The listing builds one solid part. Answer for the finished solid, in the listing's coordinates (mm). A direction names the side the tool comes from. Give positions to 0.01 mm unless a question says otherwise; leave off trailing zeros. Write each loop counter-clockwise with the first axis right and the second up, starting at its lowest first coordinate (ties: lowest second). Pieces come first, ordered by that corner, then holes. Notation, with made-up numbers: (-34, 6.5) - (-14, 6.5) arc R16 ccw to (-14, 22.5) - close; hole circle Ø5 at (60, 23). An arc over 180 degrees is marked (long way). One line per item, written item: value. Start each with the question number.
from build123d import *

# Parameters (mm, degrees)
F1_DEPTH    = 254
F2_R        = 1.5875
F3_T1_DEPTH = 511.5860222341
F3_T3_DEPTH = 513.2602424874


# Not quite as in the source:
# - a fillet or chamfer that OpenCascade refuses, or shapes differently, is made with other operations: its cross-section is extruded or revolved along the edge and cut away or added


with BuildPart() as f1:
    # F0 (on Front) → F1 (new body, symmetric)
    with BuildSketch(Plane.XZ):
        with BuildLine():
            Line((0, 16.6624), (0, 0))
            Line((0, 0), (41.275, 0))
            Line((41.275, 0), (41.275, 16.6624))
            ThreePointArc((41.275, 16.6624), (37.3126, 20.6248), (33.3502, 16.6624))
            Line((33.3502, 16.6624), (34.9377, 16.6624))
            ThreePointArc((34.9377, 16.6624), (37.3126, 19.0373), (39.6875, 16.6624))
            Line((39.6875, 16.6624), (39.6875, 1.5875))
            Line((39.6875, 1.5875), (1.5875, 1.5875))
            Line((1.5875, 1.5875), (1.5875, 16.6624))
            Line((1.5875, 16.6624), (0, 16.6624))
        make_face()
        with BuildLine():
            ThreePointArc((7.9248, 16.6624), (3.9624, 20.6248), (0, 16.6624))
            Line((0, 16.6624), (1.5875, 16.6624))
            ThreePointArc((1.5875, 16.6624), (3.9624, 19.0373), (6.3373, 16.6624))
            Line((6.3373, 16.6624), (7.9248, 16.6624))
        make_face()
    extrude(amount=F1_DEPTH, both=True)

    # F2
    f2_edges = [f1.edges().sort_by_distance(p)[0] for p in [
        (0, 0, 0),
        (41.275, 0, 0),
        (39.6875, 0, 1.5875),
        (1.5875, 0, 1.5875),
    ]]
    fillet(f2_edges, radius=F2_R)

    # F3: fillet of radius 0.8255 on 4 edges, made by hand

    # F3_s2 → F3_t1 (cut)
    with BuildSketch(Plane.XZ.offset(-255.793011117)):
        with BuildLine():
            ThreePointArc((34.2204955532, 16.6624), (34.723327211, 16.8332164322), (35.0180621764, 17.2749734127))
            ThreePointArc((35.0180621764, 17.2749734127), (34.957876249, 16.9713110978), (34.9377, 16.6624))
            Line((34.9377, 16.6624), (34.2204955532, 16.6624))
        make_face()
        with BuildLine():
            ThreePointArc((7.0545044468, 16.6624), (6.551672789, 16.8332164322), (6.2569378236, 17.2749734127))
            ThreePointArc((6.2569378236, 17.2749734127), (6.317123751, 16.9713110978), (6.3373, 16.6624))
            Line((6.3373, 16.6624), (7.0545044468, 16.6624))
        make_face()
    extrude(amount=F3_T1_DEPTH, mode=Mode.SUBTRACT)

    # F3_s4 → F3_t3 (cut)
    with BuildSketch(Plane.XZ.offset(-256.6301212437)):
        with BuildLine():
            ThreePointArc((33.4898635929, 17.7051368421), (33.6302261346, 16.9868405041), (34.2862670111, 16.6624))
            Line((34.2862670111, 16.6624), (33.3502, 16.6624))
            ThreePointArc((33.3502, 16.6624), (33.385271105, 17.1884242487), (33.4898635929, 17.7051368421))
        make_face()
        with BuildLine():
            ThreePointArc((7.7851364071, 17.7051368421), (7.6447738654, 16.9868405041), (6.9887329889, 16.6624))
            Line((6.9887329889, 16.6624), (7.9248, 16.6624))
            ThreePointArc((7.9248, 16.6624), (7.889728895, 17.1884242487), (7.7851364071, 17.7051368421))
        make_face()
    extrude(amount=F3_T3_DEPTH, mode=Mode.SUBTRACT)


solid = f1.part
Item 1: Find section A-A on z = 11.5. Determine the outline of the cut face in (x, y) (1 decimal), plus the area to 3 significant figures.
Item 2: Each of these flat-tipped pins is pushed along its axis until it touches: pin 1 Ø1 at (x, y) = (28, 17) entering from +Z; pin 2 Ø17.5 at (x, y) = (27, -68.5) entering from +Z; pin 3 Ø12 at (x, z) = (8.5, 7) entering from -Y. Where does it stop, or does it pass through?
Item 3: Find section B-B on y = -5.5. Determine the outline of the cut face in (x, z) (1 decimal).
Item 4: For faces 1 (the flat face through (0, -4, 9)), 2 (the flat face through (39.688, -4, 10)), determine the directions among +Z, -Z, +X, -X, +Y, -Y from which every point of the face is accessible in a straight line to the end or side of a thin tool.
Item 5: The mould has two halves that part along X. Classify faces 3 (the flat face through (41.275, -4, 9)), 4 (the flat face through (21, -254, 1)), 5 (the flat face through (1.588, -4, 10)): +X half, -X half, draft (parallel to the pull), parting line (faces both ways), or undercut.
Item 6: Straight lines are drawn through the part: line 1 along X through (y, z) = (123, 9.5) (1 decimal); line 2 along Z through (x, y) = (3.5, 138); line 3 along Z through (x, y) = (26.5, -174.5). For each, find the intervals that lie inside material, in ascending order.
Item 7: Find section C-C on x = 15.5. Determine the outline of the cut face in (y, z).
Values:
1. outline: (0, -254) - (1.6, -254) - (1.6, 254) - (0, 254) - close; (39.7, -254) - (41.3, -254) - (41.3, 254) - (39.7, 254) - close
1. area: 1,610 mm^2
2. pin 1: z = 1.59
2. pin 2: z = 20.3
2. pin 3: y = -254
3. outline: (0, 1.6) arc R1.6 ccw to (1.6, 0) - (39.7, 0) arc R1.6 ccw to (41.3, 1.6) - (41.3, 16.7) arc R4 ccw to (33.5, 17.7) arc R0.8 ccw to (34.3, 16.7) arc R0.8 ccw to (35, 17.3) arc R2.4 cw to (39.7, 16.7) - (39.7, 3.2) arc R1.6 cw to (38.1, 1.6) - (3.2, 1.6) arc R1.6 cw to (1.6, 3.2) - (1.6, 16.7) arc R2.4 cw to (6.3, 17.3) arc R0.8 ccw to (7, 16.7) arc R0.8 ccw to (7.8, 17.7) arc R4 ccw to (0, 16.7) - close
4. face 1: +Z, -Z, -X, +Y, -Y
4. face 2: +Y, -Y
5. face 3: +X half
5. face 4: draft
5. face 5: undercut
6. line 1: 0 to 1.6, 39.7 to 41.3
6. line 2: 0 to 1.59, 18.99 to 20.6
6. line 3: 0 to 1.59
7. outline: (-254, 0) - (254, 0) - (254, 1.59) - (-254, 1.59) - close
